from build123d import *

# Parameters (mm, degrees)
FILLET1_R = 8
FILLET2_R = 8


with BuildPart() as part:
    # Sketch1 → Revolve8 (revolve)
    with BuildSketch(Plane.XY):
        Polygon((-8.566656945, 48.024560211), (8.566656945, 48.024560211), (10, 39.895667803), (-10, 39.895667803), align=None)
    revolve(axis=Axis((0, 0, 0), (1, 0, 0)))

    # Fillet1
    fillet1_edges = [part.edges().sort_by_distance(p)[0] for p in [
        (-8.566656945, -48.024560211, 0),
    ]]
    fillet(fillet1_edges, radius=FILLET1_R)

    # Fillet2
    fillet2_edges = [part.edges().sort_by_distance(p)[0] for p in [
        (8.566656945, -48.024560211, 0),
    ]]
    fillet(fillet2_edges, radius=FILLET2_R)


solid = part.part
Work out the finished part from the listing and answer in its coordinate system (mm). Give positions to 0.01 mm unless a question says otherwise; leave off trailing zeros. One line per item, written item: value. Start each with the question number.
1. For a pull along Y with two mould halves and no side action, classify faces 1 (the cylindrical face through (-0.14, -8.649, -38.947)), 2 (the cylindrical face through (0.026, -10.411, -46.883)) as +Y half, -Y half, draft (parallel to the pull), parting line (faces both ways), or undercut.
2. Given pin 1 (3 mm diameter, centred on x = -4, y = 10, fed in from +Z); pin 2 (12 mm diameter, centred on x = -2.5, y = 14.5, fed in from -Z); pin 3 (4 mm diameter, centred on x = -5.5, y = -26.5, fed in from +Z), each flat-ended and moving along its own axis, determine where each tip first touches the part or whether it passes through.
3. Consider probe 1 along Z at (x, y) = (-0.25, 0); probe 2 along Z at (x, y) = (-6.75, -16.5); probe 3 along Y at (x, z) = (-6.5, -18). Determine where each line is inside the solid, lowest interval first.
Geometry results:
1. face 1: undercut
1. face 2: parting line
2. pin 1: z = 47.11
2. pin 2: z = -47.26
2. pin 3: z = 40.62
3. probe 1: -48.02 to -39.9, 39.9 to 48.02
3. probe 2: -43.32 to -36.32, 36.32 to 43.32
3. probe 3: -42.92 to -35.6, 35.6 to 42.92
